Part model, mm, in its own coordinate system. A direction names the side the tool comes from. Give positions to 0.01 mm unless a question says otherwise; leave off trailing zeros. Order: outer loops, then holes, each group sorted by start corner. A loop starts at its lowest first (then second) coordinate and runs counter-clockwise, first axis right, second up. Notation, with made-up numbers: (46, -21) -> (101, -21) arc R8 cw to (101, -9) -> close; hole circle Ø6 at (40, 42.5). An arc over 180 degrees is marked (long way). Write item = value, one per line. Start each with the question number.
(1) Probe line 1 along X through (y, z) = (-1.7, 18); line 2 along X through (y, z) = (-0.05, 3.5). List the from-to ranges inside material, lowest first. Write a range as from..to.
(2) Flat gauge pin, fed straight in: pin 1 (1.5 mm diameter, centred on y = -1, z = 37, fed in from -X). Where does the tip first touch, or does it go through?
(3) Saw through at B-B, the plane x = 2. List the corners of the cut face in (y, z).
(4) Which spindle directions (+Z, -Z, +X, -X, +Y, -Y) get a long thin tool onto all of the face, cutting with end or side? Do faces 4 (the flat face through (-7, -1, 7)), 5 (the flat face through (5.205, -1.479, 6.409)), 6 (the flat face through (-7, -1, 23)), 7 (the flat face through (-3, -3, 13)), 8 (the flat face through (-3, 0, 13)). Say none if no direction does.
(5) Saw through at A-A, the plane z = 32. List the corners of the cut face in (x, y).
(6) Two-plate mould, pull along Z, no slides. Class faces 1 (the flat face through (-7, -1, 37)), 2 (the flat face through (-3.24, -1.48, 36.57)), 3 (the flat face through (0.956, -1.479, 21.586)): pulls with the +Z half, pulls with the -Z half, needs draft (parallel to the pull), parting line crosses it, or undercut.
from build123d import *

# Parameters (mm, degrees)
F0_R     = 0.85
F1_DEPTH = 3


with BuildPart() as f1:
    # F0 (on Front) → F1 (new body)
    with BuildSketch(Plane.XZ):
        with BuildLine():
            ThreePointArc((-7, 16.5), (-8.5, 15), (-7, 13.5))
            Line((-7, 13.5), (-7, 14.5))
            ThreePointArc((-7, 14.5), (-7.5, 15), (-7, 15.5))
            Line((-7, 15.5), (-7, 16.5))
        make_face()
        with BuildLine():
            ThreePointArc((-7, 31.5), (-8.5, 30), (-7, 28.5))
            Line((-7, 28.5), (-7, 29.5))
            ThreePointArc((-7, 29.5), (-7.5, 30), (-7, 30.5))
            Line((-7, 30.5), (-7, 31.5))
        make_face()
        with BuildLine():
            Line((3.09036608, 13.9629782859), (3.3599960055, 13.0000142661))
            ThreePointArc((3.3599960055, 13.0000142661), (4.1506802593, 13.5380021699), (4.4555511172, 14.4444602957))
            ThreePointArc((4.4555511172, 14.4444602957), (3.862009243, 15.6395894378), (2.5511062289, 15.8889063253))
            Line((2.5511062289, 15.8889063253), (2.8207361544, 14.9259423056))
            ThreePointArc((2.8207361544, 14.9259423056), (3.2577038258, 14.8428366764), (3.4555511172, 14.4444602957))
            ThreePointArc((3.4555511172, 14.4444602957), (3.3539274979, 14.1423075871), (3.09036608, 13.9629782859))
        make_face()
        with BuildLine():
            Line((-0.9540828028, 28.4074385816), (-0.6844528773, 27.4444745619))
            ThreePointArc((-0.6844528773, 27.4444745619), (0.1062313765, 27.9824624656), (0.4111022344, 28.8889205914))
            ThreePointArc((0.4111022344, 28.8889205914), (-0.1824396398, 30.0840497335), (-1.4933426539, 30.333366621))
            Line((-1.4933426539, 30.333366621), (-1.2237127284, 29.3704026013))
            ThreePointArc((-1.2237127284, 29.3704026013), (-0.786745057, 29.2872969721), (-0.5888977656, 28.8889205914))
            ThreePointArc((-0.5888977656, 28.8889205914), (-0.6905213849, 28.5867678828), (-0.9540828028, 28.4074385816))
        make_face()
        with BuildLine():
            ThreePointArc((5.9821958457, 3.6350148368), (-1.8874094786, 6.740748138), (-7, 0))
            ThreePointArc((-7, 0), (0, -7), (7, 0))
            Line((7, 0), (5.9821958457, 3.6350148368))
        make_face()
        Circle(F0_R, mode=Mode.SUBTRACT)
        with BuildLine():
            Line((-7, 14.5), (-7, 13.5))
            ThreePointArc((-7, 13.5), (-5.9393398282, 13.9393398282), (-5.5, 15))
            ThreePointArc((-5.5, 15), (-5.9393398282, 16.0606601718), (-7, 16.5))
            Line((-7, 16.5), (-7, 15.5))
            ThreePointArc((-7, 15.5), (-6.6464466094, 15.3535533906), (-6.5, 15))
            ThreePointArc((-6.5, 15), (-6.6464466094, 14.6464466094), (-7, 14.5))
        make_face()
        with BuildLine():
            Line((-7, 29.5), (-7, 28.5))
            ThreePointArc((-7, 28.5), (-5.9393398282, 28.9393398282), (-5.5, 30))
            ThreePointArc((-5.5, 30), (-5.9393398282, 31.0606601718), (-7, 31.5))
            Line((-7, 31.5), (-7, 30.5))
            ThreePointArc((-7, 30.5), (-6.6464466094, 30.3535533906), (-6.5, 30))
            ThreePointArc((-6.5, 30), (-6.6464466094, 29.6464466094), (-7, 29.5))
        make_face()
        with BuildLine():
            ThreePointArc((2.5511062289, 15.8889063253), (1.5111050876, 14.0400154074), (3.3599960055, 13.0000142661))
            Line((3.3599960055, 13.0000142661), (3.09036608, 13.9629782859))
            ThreePointArc((3.09036608, 13.9629782859), (2.4740691073, 14.309645333), (2.8207361544, 14.9259423056))
            Line((2.8207361544, 14.9259423056), (2.5511062289, 15.8889063253))
        make_face()
        with BuildLine():
            ThreePointArc((-1.4933426539, 30.333366621), (-2.5333437952, 28.4844757031), (-0.6844528773, 27.4444745619))
            Line((-0.6844528773, 27.4444745619), (-0.9540828028, 28.4074385816))
            ThreePointArc((-0.9540828028, 28.4074385816), (-1.5703797755, 28.7541056287), (-1.2237127284, 29.3704026013))
            Line((-1.2237127284, 29.3704026013), (-1.4933426539, 30.333366621))
        make_face()
        with BuildLine():
            Line((-7, 13.5), (-7, 0))
            ThreePointArc((-7, 0), (-1.8874094786, 6.740748138), (5.9821958457, 3.6350148368))
            Line((5.9821958457, 3.6350148368), (3.3599960055, 13.0000142661))
            ThreePointArc((3.3599960055, 13.0000142661), (1.5111050876, 14.0400154074), (2.5511062289, 15.8889063253))
            Line((2.5511062289, 15.8889063253), (-0.6844528773, 27.4444745619))
            ThreePointArc((-0.6844528773, 27.4444745619), (-2.5333437952, 28.4844757031), (-1.4933426539, 30.333366621))
            Line((-1.4933426539, 30.333366621), (-5.0370359803, 42.9894142153))
            ThreePointArc((-5.0370359803, 42.9894142153), (-6.1360808221, 43.7104820287), (-7, 42.7197842898))
            Line((-7, 42.7197842898), (-7, 31.5))
            ThreePointArc((-7, 31.5), (-5.9393398282, 31.0606601718), (-5.5, 30))
            ThreePointArc((-5.5, 30), (-5.9393398282, 28.9393398282), (-7, 28.5))
            Line((-7, 28.5), (-7, 16.5))
            ThreePointArc((-7, 16.5), (-5.9393398282, 16.0606601718), (-5.5, 15))
            ThreePointArc((-5.5, 15), (-5.9393398282, 13.9393398282), (-7, 13.5))
        make_face()
    extrude(amount=F1_DEPTH)


solid = f1.part
Results list:
q1.line_1 = -7..1.96
q1.line_2 = -7..6.02
q2.pin_1 = -7
q3.outline = (-3, -6.71) -> (0, -6.71) -> (0, 17.86) -> (-3, 17.86) -> close
q4.face_4 = -Z, -X, +Y, -Y
q4.face_5 = +X, +Y, -Y
q4.face_6 = -X, +Y, -Y
q4.face_7 = +Z, -Z, +X, -X, -Y
q4.face_8 = +Z, -Z, +X, -X, +Y
q5.outline = (-7, -3) -> (-1.96, -3) -> (-1.96, 0) -> (-7, 0) -> close
q6.face_1 = needs draft
q6.face_2 = pulls with the +Z half
q6.face_3 = undercut
